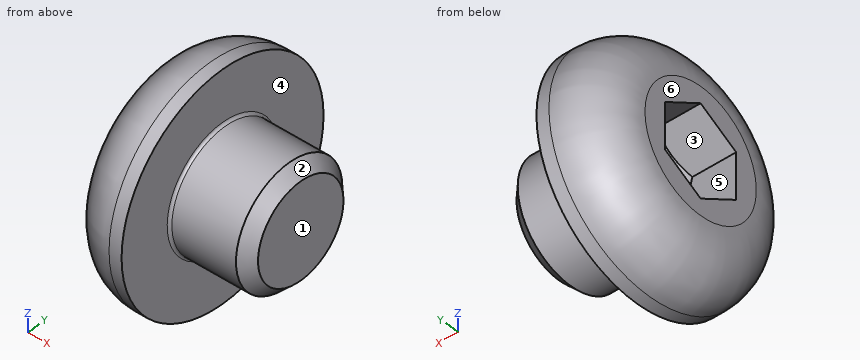
Autodesk Inventor part; units mm, degrees
ref_plane "Work Plane1" through (29, 0, 0) normal (0, -1, 0) x (1, 0, 0)
ref_plane "YZ Plane" through (0, 0, 0) normal (1, 0, 0) x (0, 1, 0)
ref_plane "XZ Plane" through (0, 0, 0) normal (0, 1, 0) x (-1, 0, 0)
sketch "Sketch1" plane through (0, 0, 0) normal (0, 0, 1) x (1, 0, 0)
  line L0 (0.2879, 0) -> (3.175, 0)
  line L1 (3.175, 0) -> (3.175, 2.413)
  line L2 (3.175, 2.413) -> (2.1084, 2.413)
  line L3 (2.1084, 2.413) -> (0.0001, 2.413)
  line L4 (0.0001, 2.413) -> (0, 2.413)
  line L5 (0, 2.413) -> (0, 4.5847)
  line L6 (0, 4.5847) -> (-2.5654, 4.5847)
  line L7 (-2.5654, 4.5847) -> (-2.5654, 1.8624)
  line L8 (-2.5654, 1.8624) -> (-0.7874, 1.8624)
  line L9 (-0.7874, 1.8624) -> (0.2879, 0)
  line L10 (-3.7135, 0) -> (4.3231, 0)
  line L11 (0, -0.9169) -> (0, 5.5016)
  line L12 (2.1084, 2.413) -> (0, 2.413) construction
  dimension "d1" = 1.0666
  dimension "d2" = 2.1083
  dimension "d3" = 2.5654
  dimension "d4" = 1.778
  dimension "d5" = 60
  dimension "d6" = 4.826
  dimension "d7" = 4.826
  dimension "d8" = 3.7248
  dimension "d9" = 9.1694
  dimension "d26" = 3.175
revolve "Body" add sketch "Sketch1" angle 360 about axis through (0.2879, 0, 0) along (1, 0, 0) contours L9 L11 L3 L2 L1 L0 | L9 L8 L7 L6 L5 L11
sketch "Sketch2" plane through (-2.5654, 0, 0) normal (-1, 0, 0) x (0, 0, 1)
  circle A0 centre (0, 0) radius 1.8624
  line L0 (0, -6.4186) -> (0, 6.4186)
  line L1 (-6.4186, 0) -> (6.4186, 0)
  line L2 (1.8624, 0) -> (0.9312, -1.6129)
  line L3 (0.9312, -1.6129) -> (-0.9312, -1.6129)
  line L4 (-0.9312, -1.6129) -> (-1.8624, 0)
  line L5 (-1.8624, 0) -> (-0.9312, 1.6129)
  line L6 (-0.9312, 1.6129) -> (0.9312, 1.6129)
  line L7 (0.9312, 1.6129) -> (1.8624, 0)
extrude "Slot" add sketch "Sketch2" against normal up to next contours L7 A0 | A0 L2 | L6 L0 A0 | A0 L0 L3 | L0 L6 A0 | A0 L3 L0 | L4 A0 | A0 L5
fillet "Fillet1" radius 2.0574 1 edges at (-2.5654, -4.5847, 0)
thread "Thread"
chamfer "Chamfer1" distance 0.4724 distance2 0.4724 1 edges at (3.175, -2.413, 0) measured on face at (3.175, -0.9842, 0.5798)
ref_plane "Work Plane1" through (29, 0, 0) normal (0, -1, 0) x (1, 0, 0)
fillet "Fillet2" radius 0.1 1 edges at (0.0001, -2.413, 0)
equation "\"d30\" = R"
equation "\"d17\" = RR"
equation "\"d13\" = GEL"
equation "\"d15\" = -0.5 * SPD + 0.5 * GD"
equation "\"d16\" = GUL"
equation "\"d1\" = GEL"
equation "\"d3\" = KOH"
equation "\"d4\" = INTI"
equation "\"d6\" = GD"
equation "\"d7\" = BDM"
equation "\"d8\" = 1.1547 * SW"
equation "\"d9\" = KOD"
equation "\"d26\" = NLG"
equation "\"GD\" = NND"
equation "\"NLG\" = 3.175"
equation "\"GEL\" = 1.0666"
equation "\"KOD\" = 9.1694"
equation "\"KOH\" = 2.5654"
equation "\"INTI\" = 1.778"
equation "\"GAL\" = 2.1082"
equation "\"GUL\" = 0.47244"
equation "\"BDM\" = NND"
equation "\"SW\" = 3.2258"
equation "\"RR\" = 2.0574"
equation "\"SPD\" = 3.88112"
equation "\"R\" = 0.1"
equation "\"TOA\" = 30deg"
equation "\"GD1\" = SPD"
equation "\"THREADDIA\" = 4.826"
equation "\"KOH1\" = 0.508"
equation "\"NND\" = 4.826"
equation "\"E0\" = 3.72593"
properties part number "ANSI B18.3 - No. 10-32 - 1/8, HSBHCSI" material "Steel, Mild"
The model under review builds one solid part; all positions refer to its coordinate system, in mm. Face numbers are marked on the shaded views. A direction names the side the tool comes from. Round coordinates to 2 decimals unless told otherwise and drop trailing zeros. Write each loop counter-clockwise with the first axis right and the second up, starting at its lowest first coordinate (ties: lowest second). Pieces come first, ordered by that corner, then holes. Notation, with made-up numbers: (68, 16) -> (99, 16) arc R36 cw to (99, 55) -> close; hole circle Ø11 at (53, 7). An arc over 180 degrees is marked (long way). Use CSV: the item, a comma, the result in double quotes.
Q1. Mouldability with a two-part tool opening along Z and no side actions: class the marked faces 1, 2 and 3 as released by +Z, released by -Z, zero draft, split by the parting line, or undercut.
Checks:
face 1,"zero draft"
face 2,"split by the parting line"
face 3,"undercut"
Q2. Consider section A-A (x = 0.95). Give the boundary of the cut face in (y, z), then the cut area to 3 significant figures.
Checks:
outline,"circle Ø4.83 at (0, 0)"
area,"18.3 mm²"
Q3. For the marked faces 4, 5 and 6, list the 3-axis set-ups (+Z, -Z, +X, -X, +Y, -Y) from which the entire face can be reached by the end or side of a thin tool; tool diameter is ignored.
Checks:
face 4,"+X"
face 5,"-X"
face 6,"+Z, -Z, -X, +Y, -Y"
Q4. To check wall thickness, follow probe 1 along Z at (x, y) = (-1.5, -1.5); probe 2 along Z at (x, y) = (-0.75, 0.25); probe 3 along Y at (x, z) = (2.9, -1). State the ranges of each line that lie inside material, in increasing order. Write a range as [from, to].
Checks:
probe 1,"[-4.06, -1], [1, 4.06]"
probe 2,"[-4.56, -1.72], [1.72, 4.56]"
probe 3,"[-1.98, 1.98]"
Q5. For pin 1 Ø0.9 at (x, z) = (-2, 0) entering from +Y; pin 2 Ø1 at (y, z) = (3, -2) entering from -X; pin 3 Ø1.5 at (x, z) = (-2, 0) entering from -Y; pin 4 Ø4 at (y, z) = (3.5, 1) entering from +X (3 decimals), all flat-tipped, find the tip position at first contact; note any pin that passes through.
Checks:
pin 1,"y = 4.3"
pin 2,"x = -2.48"
pin 3,"y = -4.45"
pin 4,"x = 3.175"
